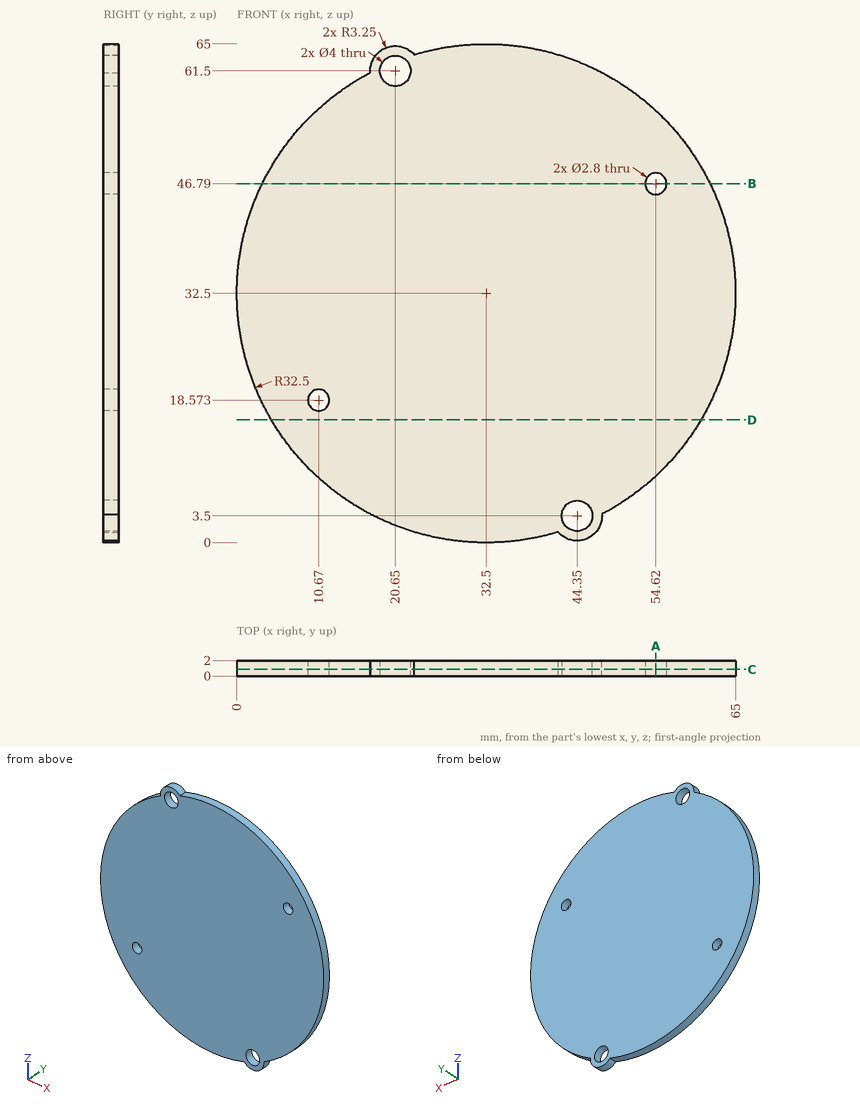
Could you check a few things on this drawing? It's one solid part, dimensions in mm from its lowest x, y, z. Round coordinates to 2 decimals unless told otherwise and drop trailing zeros. Loops run counter-clockwise (first coordinate to the right, second up) from the corner with the lowest first, then second, coordinate; pieces in that order, holes last. Notation, with made-up numbers: M 79,74.5 L 92,74.5 A18 cw 92,80.5 Z; hole C 25,29 d9. An arc over 180 degrees is marked long. Write item = value, one per line. Start each with the question number.
(1) I need wall thicknesses on line 1 along Z through (x, y) = (46, 1.2) (1 decimal); line 2 along X through (y, z) = (1.6, 46.79); line 3 along X through (y, z) = (1, 19). Which ranges of each line are inside material? Lowest first, please.
(2) Suppose I cut it at D-D on z = 16. Write out the boundary of the cut face in (x, y), plus the area to 3 significant figures.
(3) Suppose I cut it at B-B on z = 46.79. Write out the boundary of the cut face in (x, y), plus the area to 3 significant figures.
(4) Suppose I cut it at A-A on x = 54.62. Write out the boundary of the cut face in (y, z).
(5) I'm going to push a flat-ended pin straight in: P1, Ø2.5, axis at x = 20.65, z = 61.5, coming from the -Y side. Where does the tip first touch, or does it pass through?
(6) Suppose I cut it at C-C on y = 0.85. Write out the boundary of the cut face in (x, z).
Answer block:
q1.line_1 = 0.7 to 2.4, 4.6 to 62.1
q1.line_2 = 3.31 to 53.22, 56.02 to 61.69
q1.line_3 = 2.94 to 9.34, 12 to 62.06
q2.outline = M 4.5,0 L 60.5,0 L 60.5,2 L 4.5,2 Z
q2.area = 112 mm²
q3.outline = M 3.31,0 L 53.22,0 L 53.22,2 L 3.31,2 Z; M 56.02,0 L 61.69,0 L 61.69,2 L 56.02,2 Z
q3.area = 111 mm²
q4.outline = M 0,8.69 L 2,8.69 L 2,45.39 L 0,45.39 Z; M 0,48.19 L 2,48.19 L 2,56.31 L 0,56.31 Z
q5.P1 = through
q6.outline = M 17.41,61.28 A32.5 ccw 41.88,1.38 A3.25 ccw 47.59,3.72 A32.5 ccw 23.12,63.62 A3.25 ccw Z; hole C 10.67,18.57 d2.8; hole C 20.65,61.5 d4; hole C 44.35,3.5 d4; hole C 54.62,46.79 d2.8
